Input: dimensioned drawing with shaded views. Units: mm. Origin: part minimum x, y, z. Coordinates: 2 decimals unless noted, no trailing zeros. Loops run counter-clockwise (first coordinate to the right, second up) from the corner with the lowest first, then second, coordinate; pieces in that order, holes last.
Item 1: Section B-B on z = 13.5. Return loops of the section in (x, y) (1 decimal).
Item 2: Section C-C on y = 13.25. Return loops of the section in (x, z).
Item 3: Pull-direction query (X, two-part tool) for the marked faces 1, 2 and 3; classes: released by +X, released by -X, zero draft, split by the parting line, or undercut.
Item 4: Section D-D on x = 4. Return loops of the section in (y, z).
Item 5: Contact query for flat-ended pins moving along their axis: P1, Ø5, axis at x = 15.5, z = 10.5, coming from the +Y side; P2, Ø1.5, axis at x = 27, y = 11.5, coming from the -Z side; P3, Ø5, axis at y = 7.5, z = 5.5, coming from the +X side (1 decimal); P4, Ø5, axis at x = 10.5, y = 8.5, coming from the -Z side. Output: stop coordinate, or through.
Item 6: Section A-A on x = 15. Return loops of the section in (y, z), and give its area (3 significant figures).
Item 7: Ray query, line 1 along Z through (x, y) = (15, 6.25); line 2 along X through (y, z) = (6.75, 15); line 3 along X through (y, z) = (11.75, 15) (1 decimal). Return the intervals inside material, ascending.
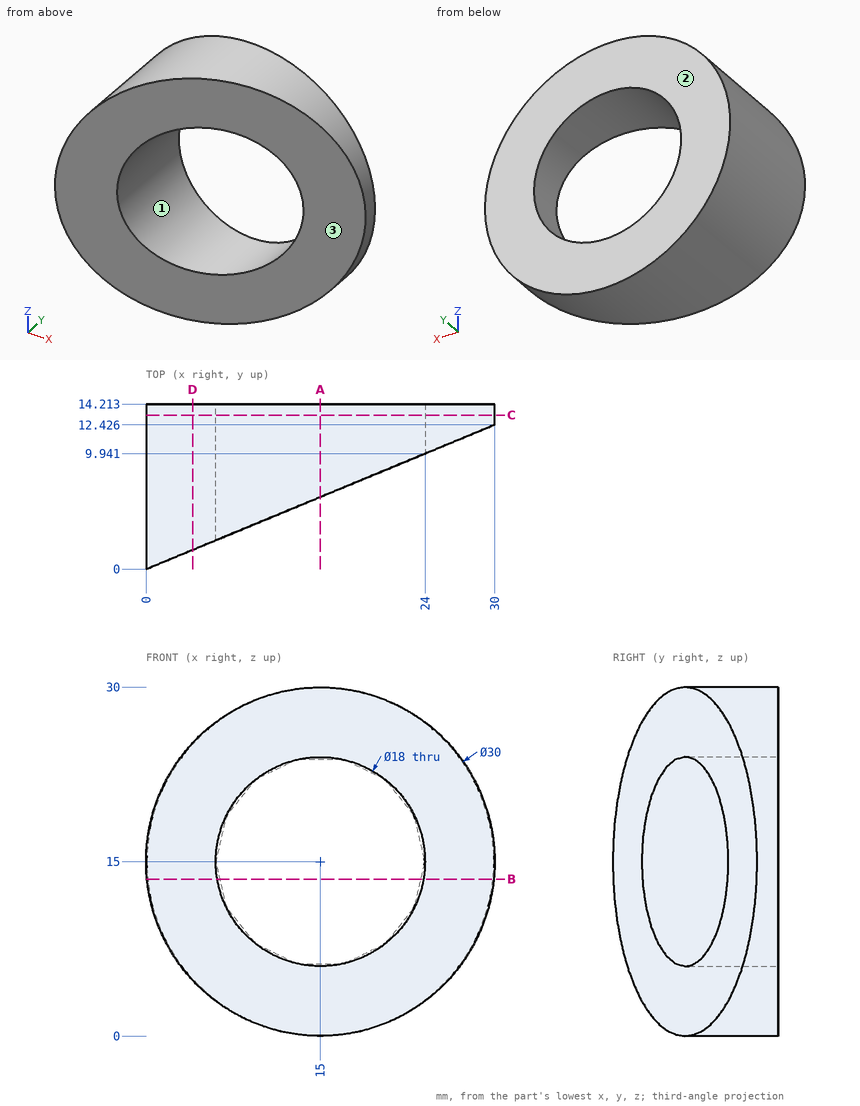
Results found:
1. outline: (0.1, 0) - (6.1, 2.5) - (6.1, 14.2) - (0.1, 14.2) - close; (23.9, 9.9) - (29.9, 12.4) - (29.9, 14.2) - (23.9, 14.2) - close
2. outline: circle Ø30 at (15, 15); hole circle Ø18 at (15, 15)
3. face 1: undercut
3. face 2: zero draft
3. face 3: released by +X
4. outline: (1.66, 4.8) - (14.21, 4.8) - (14.21, 25.2) - (1.66, 25.2) - close
5. P1: passes through
5. P2: stops at z = 5.08
5. P3: stops at x = 24.1
5. P4: stops at z = 0.13
6. outline: (6.21, 0) - (14.21, 0) - (14.21, 6) - (6.21, 6) - close; (6.21, 24) - (14.21, 24) - (14.21, 30) - (6.21, 30) - close
6. area: 96.0 mm2
7. line 1: z = 0 to 6, 24 to 30
7. line 2: x = 0 to 6
7. line 3: x = 0 to 6, 24 to 28.4
